Read the model definition and answer for the solid it produces. Units are mm, in the model's axes. A direction names the side the tool comes from. Coordinates: 2 decimals unless noted, no trailing zeros. Loops run counter-clockwise (first coordinate to the right, second up) from the corner with the lowest first, then second, coordinate; pieces in that order, holes last. Notation, with made-up numbers: (67, -32) - (105, -32) arc R29 cw to (105, 2) - close; hole circle Ø10 at (84.25, 3). An arc over 180 degrees is marked (long way). Use one line per item in the form item = value. Start each with the question number.
1) A cutting plane is placed at A-A (z = 10). Give the vertices of the cut face in (x, y).
2) Which of the six approach directions +Z, -Z, +X, -X, +Y, -Y give full straight-line access (tool end or side, diameter ignored) to faces 1 (the face through (-65, -1, 7.5)), 2 (the face through (-39, 1, 0)), 3 (the face through (-65, -1, 12.5)), 4 (the face through (-77.5, -1.5, 9.9)), 5 (the face through (-39, 1, 20))?
3) A cutting plane is placed at C-C (x = -81.5). Give the vertices of the cut face in (y, z), and give its area (3 significant figures).
4) Consider line 1 (Z direction, x = -8, y = 0.25); line 2 (X direction, y = -5, z = 7); line 3 (X direction, y = -2.75, z = 11.5). Determine where each line is inside the solid, lowest interval first.
5) A cutting plane is placed at B-B (y = 1.5). Give the vertices of the cut face in (x, z).
6) Each of these flat-tipped pins is pushed along its axis until it touches: P1, Ø6.5, axis at x = -56, y = -2, coming from the +Z side; P2, Ø1.5, axis at y = -2.5, z = 46.5, coming from the -X side; P3, Ø1.5, axis at x = -64.5, y = -2, coming from the -Z side; P4, Ø1.5, axis at x = -70, y = -1.5, coming from the +Z side. Where does it stop, or does it pass through?
from build123d import *

# Parameters (mm, degrees)
SKETCH1_W           = 120
SKETCH1_H           = 20
BOSS_EXTRUDE1_DEPTH = 3
SKETCH2_W           = 20
SKETCH2_H           = 13
BOSS_EXTRUDE2_DEPTH = 3
BOSS_EXTRUDE3_DEPTH = 3
BOSS_EXTRUDE4_DEPTH = 3


with BuildPart() as part:
    # Sketch1 → Boss-Extrude1 (new body)
    with BuildSketch(Plane(origin=(0, 0, 0), x_dir=(1, 0, 0), z_dir=(0, 1, 0))):
        with Locations((-60, -10)):
            Rectangle(SKETCH1_W, SKETCH1_H)
    extrude(amount=BOSS_EXTRUDE1_DEPTH)

    # Sketch2 → Boss-Extrude2 (add)
    with BuildSketch(Plane(origin=(0, 0, 0), x_dir=(0, 0, -1), z_dir=(1, 0, 0))):
        with Locations((-10, -3.5)):
            Rectangle(SKETCH2_W, SKETCH2_H)
    extrude(amount=BOSS_EXTRUDE2_DEPTH)

    # Sketch3 → Boss-Extrude3 (add)
    with BuildSketch(Plane(origin=(0, 3, 0), x_dir=(1, 0, 0), z_dir=(0, 1, 0))):
        with BuildLine():
            Line((-120, -20), (-120, -58.131635164))
            ThreePointArc((-120, -58.131635164), (-118.492697657, -60.069997622), (-116.242750981, -59.086661805))
            Line((-116.242750981, -59.086661805), (-95, -20))
            Line((-95, -20), (-120, -20))
        make_face()
        with BuildLine():
            Line((-120, 0), (-120, 38.131635164))
            ThreePointArc((-120, 38.131635164), (-118.492697657, 40.069997622), (-116.242750981, 39.086661805))
            Line((-116.242750981, 39.086661805), (-95, 0))
            Line((-95, 0), (-120, 0))
        make_face()
    extrude(amount=-BOSS_EXTRUDE3_DEPTH)

    # Sketch5 → Boss-Extrude4 (add)
    with BuildSketch(Plane.XZ):
        with BuildLine():
            Line((-55, 7.5), (-75, 7.5))
            ThreePointArc((-75, 7.5), (-77.5, 10), (-75, 12.5))
            Line((-75, 12.5), (-55, 12.5))
            ThreePointArc((-55, 12.5), (-52.5, 10), (-55, 7.5))
        make_face()
    extrude(amount=BOSS_EXTRUDE4_DEPTH)


solid = part.part
Found:
q1.outline = (-120, 0) - (-77.5, 0) - (-77.5, -3) - (-52.5, -3) - (-52.5, 0) - (0, 0) - (0, -10) - (3, -10) - (3, 3) - (-120, 3) - close
q2.face_1 = -Z, -X, -Y
q2.face_2 = -Z, +X, +Y, -Y
q2.face_3 = +Z, -X, -Y
q2.face_4 = -X, -Y
q2.face_5 = +Z, +X, +Y, -Y
q3.outline = (0, 0) - (3, 0) - (3, 20) - (0, 20) - close
q3.area = 60.0 mm^2
q4.line_1 = 0 to 20
q4.line_2 = 0 to 3
q4.line_3 = -77 to -53, 0 to 3
q5.outline = (-120, -38.13) arc R2 ccw to (-116.24, -39.09) - (-95, 0) - (3, 0) - (3, 20) - (-95, 20) - (-116.24, 59.09) arc R2 ccw to (-120, 58.13) - close
q6.P1 = 20
q6.P2 = through
q6.P3 = 7.5
q6.P4 = 12.5
